```python
from build123d import *

# Parameters (mm, degrees)
SKETCH1_W           = 10
SKETCH1_H           = 11
BOSS_EXTRUDE1_DEPTH = 5
SKETCH3_W           = 5
SKETCH3_H           = 5.5
CUT_EXTRUDE1_DEPTH  = 5
SKETCH4_R           = 1.5
CUT_EXTRUDE2_DEPTH  = 5
SKETCH5_R           = 1.5
CUT_EXTRUDE3_DEPTH  = 10
FILLET1_R           = 2.5
FILLET2_R           = 2.5


with BuildPart() as part:
    # Sketch1 → Boss-Extrude1 (new body)
    with BuildSketch(Plane(origin=(0, 0, 0), x_dir=(1, 0, 0), z_dir=(0, 1, 0))):
        Rectangle(SKETCH1_W, SKETCH1_H)
    extrude(amount=BOSS_EXTRUDE1_DEPTH)

    # Sketch3 → Cut-Extrude1 (cut)
    with BuildSketch(Plane(origin=(0, 5, 0), x_dir=(1, 0, 0), z_dir=(0, 1, 0))):
        with Locations((0, -2.75)):
            Rectangle(SKETCH3_W, SKETCH3_H)
    extrude(amount=-CUT_EXTRUDE1_DEPTH, mode=Mode.SUBTRACT)

    # Sketch4 → Cut-Extrude2 (cut)
    with BuildSketch(Plane(origin=(0, 5, 0), x_dir=(1, 0, 0), z_dir=(0, 1, 0))):
        with Locations(Location((0, 3, 0), (0, 0, 270))):
            Circle(SKETCH4_R)
    extrude(amount=-CUT_EXTRUDE2_DEPTH, mode=Mode.SUBTRACT)

    # Sketch5 → Cut-Extrude3 (cut)
    with BuildSketch(Plane.ZY.offset(5)):
        with Locations((3, 2.5)):
            Circle(SKETCH5_R)
    extrude(amount=-CUT_EXTRUDE3_DEPTH, mode=Mode.SUBTRACT)

    # Fillet1
    fillet1_edges = [part.edges().sort_by_distance(p)[0] for p in [
        (3.75, 0, 5.5),
        (3.75, 5, 5.5),
        (-3.75, 0, 5.5),
        (-3.75, 5, 5.5),
    ]]
    fillet(fillet1_edges, radius=FILLET1_R - 0.0001)  # a hair under: the kernel refuses the full size

    # Fillet2
    fillet2_edges = [part.edges().sort_by_distance(p)[0] for p in [
        (-5, 2.5, -5.5),
        (5, 2.5, -5.5),
    ]]
    fillet(fillet2_edges, radius=FILLET2_R)


solid = part.part
```
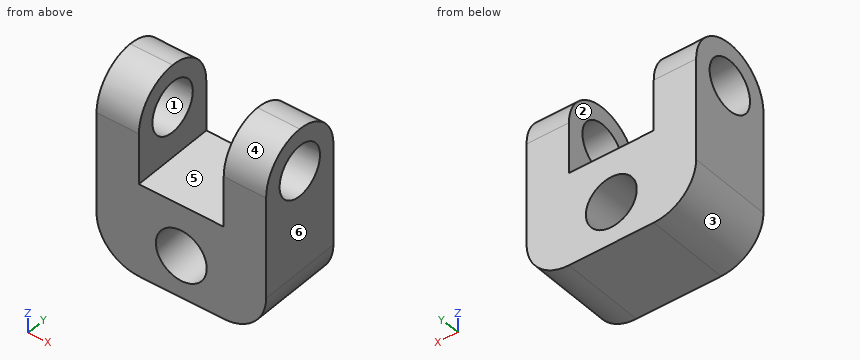
Geometry check sheet. Reference: the model listing, model coordinates, mm. Face numbers are marked on the shaded views. A direction names the side the tool comes from. Give positions to 0.01 mm unless a question says otherwise; leave off trailing zeros. Order: outer loops, then holes, each group sorted by start corner. A loop starts at its lowest first (then second) coordinate and runs counter-clockwise, first axis right, second up. Notation, with made-up numbers: (-29, 7.5) -> (-16, 7.5) arc R24 cw to (-16, 23.5) -> close; hole circle Ø10 at (18, -34). An arc over 180 degrees is marked (long way). Write each question's results on one line, items separated by ' | '. Start each with the question number.
(1) Sectioned sample at D-D (z = -2). Enter the section's corners in (x, y), plus the area to 3 significant figures.
(2) Access from +Z, -Z, +X, -X, +Y, -Y to the whole of each face (thin tool, end or side, straight path). Record for the marked faces 1 and 2.
(3) Mould release check, pull along X, two halves, no side actions. Record for the marked faces 3, 4, 5 and 6: pulls with the +X half, pulls with the -X half, needs draft (parallel to the pull), parting line crosses it, or undercut.
(4) Scan lines: line 1 (X direction, y = 1.8, z = 4.75); line 2 (X direction, y = 1.7, z = -3); line 3 (Y direction, x = 3.3, z = 3). Record each from-to range of solid material in increasing order.
(5) Gauge pin test, flat end, axial feed: P1, Ø1.5, axis at x = 0, y = 2.5, coming from the +Z side. Record the tip position at first contact, or that the pin passes through.
(6) Sectioned sample at A-A (x = 0). Enter the section's corners in (y, z).
(7) Sectioned sample at B-B (y = 2.25). Enter the section's corners in (x, z), plus the area to 3 significant figures.
Answer below:
1) outline: (-5, 0) -> (-1.12, 0) -> (-1.12, 5) -> (-5, 5) -> close; (1.12, 0) -> (5, 0) -> (5, 5) -> (1.12, 5) -> close | area: 38.8 mm2
2) face 1: +X, -X | face 2: +Z, +Y, -Y
3) face 3: pulls with the -X half | face 4: needs draft | face 5: undercut | face 6: pulls with the +X half
4) line 1: -5 to -2.5, 2.5 to 5 | line 2: -5 to -1.5, 1.5 to 5 | line 3: 0 to 1, 4 to 5
5) P1: z = 0
6) outline: (0, -5.5) -> (5, -5.5) -> (5, -4.5) -> (0, -4.5) -> close; (0, -1.5) -> (5, -1.5) -> (5, 0) -> (0, 0) -> close
7) outline: (-5, -3) arc R2.5 ccw to (-2.5, -5.5) -> (2.5, -5.5) arc R2.5 ccw to (5, -3) -> (5, 1.52) -> (2.5, 1.52) -> (2.5, 0) -> (-2.5, 0) -> (-2.5, 1.52) -> (-5, 1.52) -> close; (-5, 4.48) -> (-2.5, 4.48) -> (-2.5, 5.49) -> (-5, 5.49) -> close; (2.5, 4.48) -> (5, 4.48) -> (5, 5.49) -> (2.5, 5.49) -> close; hole circle Ø3 at (0, -3) | area: 57.9 mm2
